Read the model definition and answer for the solid it produces. Units are mm, in the model's axes. Face numbers are marked on the shaded views. A direction names the side the tool comes from. Round coordinates to 2 decimals unless told otherwise and drop trailing zeros. Loops run counter-clockwise (first coordinate to the right, second up) from the corner with the lowest first, then second, coordinate; pieces in that order, holes last. Notation, with made-up numbers: (-26, 81.5) - (30, 81.5) arc R14 cw to (30, 86.5) - close; hole circle Ø11 at (39.25, -17.5). An arc over 180 degrees is marked (long way). Answer as CSV lines item,"result".
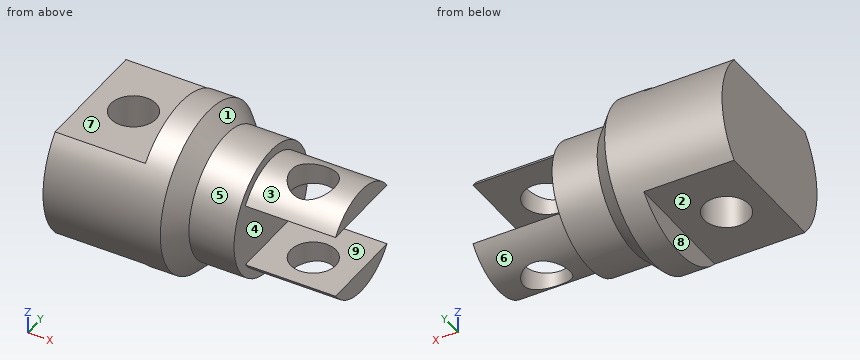
Autodesk Inventor part; units mm, degrees
ref_plane "Work Plane1" through (7.5, 0, 9) normal (0, 0, 1) x (1, 0, 0)
ref_plane "YZ Plane" through (0, 0, 0) normal (1, 0, 0) x (0, 1, 0)
ref_plane "XZ Plane" through (0, 0, 0) normal (0, 1, 0) x (-1, 0, 0)
sketch "Sketch1" plane through (0, 0, 0) normal (0, 0, 1) x (1, 0, 0)
  line L0 (0, 0) -> (30, 0)
  line L1 (0, 0) -> (0, 9)
  line L2 (0, 9) -> (15, 9)
  line L3 (15, 9) -> (15, 7)
  line L4 (15, 7) -> (20, 7)
  line L5 (20, 7) -> (20, 6)
  line L6 (20, 6) -> (30, 6)
  line L7 (30, 6) -> (30, 0)
  dimension "d5" = 18
  dimension "d6" = 5
  dimension "d7" = 14
  dimension "d8" = 12
  dimension "d9" = 10
  dimension "d10" = 15
revolve "Revolution1" add sketch "Sketch1" angle 360 about axis through (0, 0, 0) along (1, 0, 0)
chamfer "Chamfer1" distance 2 angle 45 1 edges at (15, -9, 0)
ref_plane "Work Plane1" through (7.5, 0, 9) normal (0, 0, 1) x (1, 0, 0)
sketch "Sketch2" plane through (7.5, 0, 9) normal (0, 0, 1) x (1, 0, 0)
  line L0 (-7.5, -9) -> (-7.5, 9)
  line L1 (2.5, 8) -> (-7.5, 8)
  line L2 (-7.5, 8) -> (-7.5, -12)
  line L3 (-7.5, -12) -> (2.5, -12)
  line L4 (2.5, -12) -> (2.5, 8)
  line L5 (-7.5, -9) -> (-7.5, 9)
  line L6 (-7.5, -9) -> (5.5, -9)
  line L7 (-7.5, 9) -> (5.5, 9)
  line L8 (5.5, -9) -> (5.5, 9)
  point P0 (-7.5, 0)
  point P1 (-7.5, 8)
  dimension "d11" = 10
  dimension "d14" = 20
  dimension "d15" = -1
  dimension "d16" = 3
  dimension "d19" = 18
extrude "Extrusion1" cut sketch "Sketch2" against normal blind 3 contours L6 L4 L3 L2 | L0 L1 L4 L6
mirror "Mirror1" about plane through (0, 0, 0) normal (0, 0, 1) of "Extrusion1"
sketch "Sketch3" plane through (7.5, 0, 6) normal (0, 0, 1) x (1, 0, 0)
  point P0 (-7.5, 0)
  point P1 (-2.6939, -0.0831)
hole "Hole1" at (4.8061, -0.0831, 6) direction (0, 0, -1) diameter 5 end through all
sketch "Sketch4" plane through (30, 0, 0) normal (1, 0, 0) x (0, 0, -1)
  circle A0 centre (0, 0) radius 6
  circle A1 centre (0, 0) radius 7
  circle A2 centre (0, 0) radius 6
  circle A3 centre (0, 0) radius 7
  line L0 (-3.5, 6.0622) -> (3.5, 6.0622)
  line L1 (3.5, 6.0622) -> (3.5, -6.0622)
  line L2 (3.5, -6.0622) -> (-3.5, -6.0622)
  line L3 (-3.5, -6.0622) -> (-3.5, 6.0622)
  line L4 (0, -12.6) -> (0, 12.6)
  point P0 (-3.5, -6.0622)
  point P1 (3.5, -6.0622)
  point P2 (3.5, 6.0622)
  point P3 (-3.5, 6.0622)
  dimension "d27" = 7
extrude "Extrusion2" cut sketch "Sketch4" against normal blind 10 contours L1 A0 L4 | A0 L4 L0 L1 | L1 L2 L4 A0 | L4 A0 L3 | A0 L3 L0 L4 | L0 L4 A1 | L4 L2 L3 A0 | A1 L4 L2 | L0 A1 L4 | L4 A1 L2
sketch "Sketch5" plane through (30, -4.8734, 3.5) normal (0, 0, -1) x (-1, 0, 0)
  line L0 (0, 9.7468) -> (10, 9.7468)
  line L1 (10, 9.7468) -> (10, 0)
  line L2 (10, 0) -> (0, 0)
  line L3 (0, 9.7468) -> (0, 0)
  circle A0 centre (4.9634, 4.2697) radius 2.5
  line L4 (4.9634, 4.2697) -> (0, 4.8734) construction
  line L5 (0, 9.7468) -> (0, 0)
  line L6 (4.9634, 4.2697) -> (5, 9.7468) construction
  point P0 (30, 4.8734)
  dimension "d30" = 5
  dimension "d32" = 5.4772
  dimension "d33" = 5
extrude "Extrusion3" cut sketch "Sketch5" along normal through all both and the other way through all contours A0
equation "\"d15\" = -0.5 * d14 + 0.5 * d19"
properties part number "McCrea_krk_walle"
1) A cutting plane is placed at C-C, the plane y = 0. Count the separate pieces of the cut face and the enclosed holes in it, plus the area to 3 significant figures.
Entries:
separate pieces,"4"
enclosed holes,"0"
area,"242 mm^2"
2) A cutting plane is placed at B-B, the plane x = 5.5. Determine the outline of the cut face in (y, z).
Entries:
outline,"(-6.71, -6) - (-2.48, -6) - (-2.48, 6) - (-6.71, 6) arc R9 ccw to start; (2.32, -6) - (6.71, -6) arc R9 ccw to (6.71, 6) - (2.32, 6) - close"
3) The mould has two halves that part along Z. Classify the marked faces 1, 2, 3 and 4: pulls with the +Z half, pulls with the -Z half, needs draft (parallel to the pull), parting line crosses it, or undercut.
Entries:
face 1,"parting line crosses it"
face 2,"pulls with the -Z half"
face 3,"pulls with the +Z half"
face 4,"undercut"
4) A cutting plane is placed at A-A, the plane x = 23.5. Determine the outline of the cut face in (y, z).
Entries:
outline,"(-4.87, -3.5) arc R6 ccw to (-2.58, -5.42) - (-2.58, -3.5) - close; (-4.87, 3.5) - (-2.58, 3.5) - (-2.58, 5.42) arc R6 ccw to start; (1.37, -5.84) arc R6 ccw to (4.87, -3.5) - (1.37, -3.5) - close; (1.37, 3.5) - (4.87, 3.5) arc R6 ccw to (1.37, 5.84) - close"
5) Find the intervals of material crossed by line 1 (Z direction, x = 22, y = -0.25); line 2 (Z direction, x = 6.5, y = 2); line 3 (X direction, y = -4.5, z = -2), in increasing order.
Entries:
line 1,"z = -5.99 to -3.5, 3.5 to 5.99"
line 2,"z = -6 to 6"
line 3,"x = 0 to 20"
6) A tool of negligible diameter and unlimited length cuts with its end or side. For the marked faces 5, 6, 7, 8 and 9, from which of +Z, -Z, +X, -X, +Y, -Y can it reach the whole face along a straight path? Write none if from no direction.
Entries:
face 5,"+X"
face 6,"-Z, +X"
face 7,"+Z, -X, +Y, -Y"
face 8,"-Z, -X, +Y, -Y"
face 9,"+X, +Y, -Y"
7) Each of these flat-tipped pins is pushed along its axis until it touches: P1, Ø5, axis at x = 5, y = -2.5, coming from the +Z side; P2, Ø4, axis at x = 11.5, z = -6, coming from the -Y side; P3, Ø6, axis at x = 25.04, y = -0.6, coming from the -Z side. Where does it stop, or does it pass through?
Entries:
P1,"stops at z = 6"
P2,"stops at y = -8.06"
P3,"stops at z = -6"
